```python
from build123d import *

# Parameters (mm, degrees)
SKETCH1_R           = 2.5
BOSS_EXTRUDE1_DEPTH = 11
SKETCH2_R           = 21.969303103
CUT_EXTRUDE1_DEPTH  = 8.5
BOSS_EXTRUDE2_DEPTH = 54


with BuildPart() as part:
    # Sketch1 → Boss-Extrude1 (new body, symmetric)
    with BuildSketch(Plane.XY):
        with BuildLine():
            Line((-75.294135102, -21.801947472), (-75.916524457, 0.530755))
            Line((-75.916524457, 0.530755), (-6.210315137, 21.073259471))
            ThreePointArc((-6.210315137, 21.073259471), (21.281751318, -5.453195364), (-15.579203419, -15.489954799))
            Line((-15.579203419, -15.489954799), (-75.294135102, -21.801947472))
        make_face()
        Circle(SKETCH1_R, mode=Mode.SUBTRACT)
    boss_extrude1 = extrude(amount=BOSS_EXTRUDE1_DEPTH, both=True)

    # Sketch2 → Cut-Extrude1 (cut, symmetric)
    with BuildSketch(Plane.XY):
        Circle(SKETCH2_R)
    cut_extrude1 = extrude(amount=CUT_EXTRUDE1_DEPTH, both=True, mode=Mode.SUBTRACT)

    # Sketch3 → Boss-Extrude2 (add)
    with BuildSketch(Plane(origin=(0, 0, -11), x_dir=(-1, 0, 0), z_dir=(0, 0, -1))):
        Polygon((75.294135102, -21.801947472), (75.916524457, 0.530755), (75.60532978, 0.622464449), (56.412661227, 6.278567161), (53.685919424, -19.517914062), align=None)
    boss_extrude2 = extrude(amount=BOSS_EXTRUDE2_DEPTH)

    # Mirror3: Boss-Extrude1, Cut-Extrude1, Boss-Extrude2 across plane
    add(boss_extrude1.mirror(Plane(origin=(-98.145469491, -3.551481911, -65), x_dir=(1, 0, 0), z_dir=(0, 0, 1))))
    add(cut_extrude1.mirror(Plane(origin=(-98.145469491, -3.551481911, -65), x_dir=(1, 0, 0), z_dir=(0, 0, 1))), mode=Mode.SUBTRACT)
    add(boss_extrude2.mirror(Plane(origin=(-98.145469491, -3.551481911, -65), x_dir=(1, 0, 0), z_dir=(0, 0, 1))))


solid = part.part
```
CAD build for the part. Positions are in the model's coordinates, mm. A direction names the side the tool comes from. Round coordinates to 2 decimals unless told otherwise and drop trailing zeros. Order: outer loops, then holes, each group sorted by start corner. A loop starts at its lowest first (then second) coordinate and runs counter-clockwise, first axis right, second up. Notation, with made-up numbers: (-38.5, 68) -> (-32.5, 68) arc R16 cw to (-32.5, 89) -> close; hole circle Ø2 at (25, 61.25). An arc over 180 degrees is marked (long way). Write item = value, one per line.
(1) 3-axis set-ups, long thin cutter, end or side, ignore diameter. For faces 5 (the cylindrical face through (-21.2, 5.76, 0.12)), 6 (the cylindrical face through (21.433, -4.823, 9.768)): which of +Z, -Z, +X, -X, +Y, -Y reach the whole face in a straight line?
Answers follow:
face_5 = +X
face_6 = +Z, -Z
(2) Drill centre lines: L1, parallel to Z at x = -16, y = 3; L2, parallel to Z at x = -35.5, y = -5; L3, parallel to Y at x = 0, z = -9.6. Where is each one in solid material? Low to high.
Answers follow:
L1 = -141 to -138.5, -121.5 to -119, -11 to -8.5, 8.5 to 11
L2 = -141 to -119, -11 to 11
L3 = -21.97 to -2.5, 2.5 to 21.97
(3) Cut at C-C (z = -54.5). Write the cut outline in (x, y).
Answers follow:
outline = (-75.92, 0.53) -> (-75.29, -21.8) -> (-53.69, -19.52) -> (-56.41, 6.28) -> close
(4) Cut at D-D (x = 12.5). Write the cut outline in (y, z), plus the area to 3 significant figures.
Answers follow:
outline = (-18.07, -141) -> (18.07, -141) -> (18.07, -138.5) -> (-18.07, -138.5) -> close; (-18.07, -121.5) -> (18.07, -121.5) -> (18.07, -119) -> (-18.07, -119) -> close; (-18.07, -11) -> (18.07, -11) -> (18.07, -8.5) -> (-18.07, -8.5) -> close; (-18.07, 8.5) -> (18.07, 8.5) -> (18.07, 11) -> (-18.07, 11) -> close
area = 361 mm²
(5) Cut at A-A (x = 0). State how many separate pieces and enclosed holes the cut face has, plus the area to 3 significant figures.
Answers follow:
separate_pieces = 8
enclosed_holes = 0
area = 389 mm²
(6) Cut at B-B (x = -24.5). Write the cut outline in (y, z), plus the area to 3 significant figures.
Answers follow:
outline = (-16.43, -141) -> (15.68, -141) -> (15.68, -119) -> (-16.43, -119) -> close; (-16.43, -11) -> (15.68, -11) -> (15.68, 11) -> (-16.43, 11) -> close
area = 1,410 mm²
(7) Flat gauge pin, fed straight in: P1, Ø4, axis at x = 0, y = 0, coming from the +Z side. Where does the tip first touch, or does it go through?
Answers follow:
P1 = through
(8) Pull direction Z, two halves, no side cores. Call faces 1 (the cylindrical face through (21.433, -4.823, -139.768)), 2 (the flat face through (-26, 0, -141)), 3 (the flat face through (-55.07, -6.44, -65.76)), 4 (the flat face through (5, 0, -138.5)): +Z half, -Z half, draft (parallel to the pull), parting line (faces both ways), or undercut.
Answers follow:
face_1 = draft
face_2 = -Z half
face_3 = undercut
face_4 = undercut
